Verification items for the finished model (mm, model axes). A direction names the side the tool comes from. Round coordinates to 2 decimals unless told otherwise and drop trailing zeros. Write each loop counter-clockwise with the first axis right and the second up, starting at its lowest first coordinate (ties: lowest second). Pieces come first, ordered by that corner, then holes. Notation, with made-up numbers: M -35.5,58 L -6.5,58 A25 ccw -6.5,94 Z; hole C 34,-19.75 d2. An arc over 180 degrees is marked long. One line per question, with ' | ' between items.
Autodesk Inventor part; units mm, degrees
ref_plane "YZ Plane" through (0, 0, 0) normal (1, 0, 0) x (0, 1, 0)
ref_plane "XZ Plane" through (0, 0, 0) normal (0, 1, 0) x (-1, 0, 0)
ref_plane "XY Plane" through (0, 0, 0) normal (0, 0, 1) x (1, 0, 0)
sketch "Esboço1" plane through (0, 0, 0) normal (0, 0, 1) x (1, 0, 0)
  line L0 (17.7277, 1.9549) -> (-24.2723, 1.9549)
  line L1 (-24.2723, 1.9549) -> (-24.2723, 7.9549)
  line L2 (17.7277, 7.9549) -> (17.7277, 1.9549)
  line L3 (6.7277, 39.4549) -> (6.7277, 7.9549)
  line L4 (-13.2723, 7.9549) -> (-13.2723, 39.4549)
  arc A0 (-4.2723, 30.871) -> (-2.2723, 30.871) centre (-3.2723, 24.9549) ccw
  line L5 (-24.2723, 7.9549) -> (-13.2723, 7.9549)
  line L6 (6.7277, 7.9549) -> (17.7277, 7.9549)
  line L7 (-2.2723, 39.4549) -> (-2.2723, 30.871)
  line L8 (-4.2723, 30.871) -> (-4.2723, 39.4549)
  line L9 (-13.2723, 39.4549) -> (-4.2723, 39.4549)
  line L10 (-2.2723, 39.4549) -> (6.7277, 39.4549)
  dimension "largura" = 42
  dimension "largura_topo" = 20
  dimension "altura_base" = 6
  dimension "diametro" = 12
  dimension "altura_furo" = 23
  dimension "d6" = 11
  dimension "d7" = 10
  dimension "d8" = 6
  dimension "d10" = 9
  dimension "d11" = 9
  dimension "altura" = 37.5
  dimension "d33" = 37.5
extrude "Extrusão1" add sketch "Esboço1" along normal blind 16
sketch "Esboço2" plane through (6.7277, 7.9549, 0) normal (1, 0, 0) x (0, 0, -1)
  line L0 (0, 22.9161) -> (-16, 22.9161)
  line L1 (-8, 22.9161) -> (-8, 31.5) construction
  circle A0 centre (-8, 27.208) radius 1.1711 construction
  line L2 (0, 31.5) -> (-16, 31.5)
  point P0 (0, -7.9549)
hole "Furo1" at (6.7277, 35.163, 8) direction (-1, 0, 0) diameter 3.242 end through all counterbore diameter 6 counterbore depth 4
sketch "Esboço3" plane through (-24.2723, 1.9549, 0) normal (0, -1, 0) x (1, 0, 0)
  line L0 (5, 8) -> (37, 8) construction
  circle A0 centre (5, 8) radius 1 construction
  circle A1 centre (37, 8) radius 1 construction
  line L1 (42, 0) -> (0, 0) construction
  line L2 (21, 0) -> (21, 16) construction
  line L3 (0, 16) -> (42, 16) construction
  point P0 (21, 8)
  dimension "distancia_parafusos" = 32
  dimension "d22" = 2
  dimension "d23" = 2
hole "Furo2" at (-19.2723, 1.9549, 8) at (12.7277, 1.9549, 8) direction (0, 1, 0) diameter 5.5 end through all
fillet "Arredondamento1" radius 1 4 edges at (6.7277, 39.4549, 8) (-13.2723, 39.4549, 8) (-24.2723, 7.9549, 8) (17.7277, 7.9549, 8)
equation "\"d6\" = -0.5 * largura_topo + 0.5 * largura"
equation "\"d7\" = 0.5 * largura_topo"
equation "\"d8\" = altura_base"
equation "\"d11\" = d10"
equation "\"d33\" = altura"
properties part number "Sk12"
1. Section check C-C, the plane z = 4.5. Record the cut outline in (x, y).
Results:
outline: M -24.27,1.95 L 17.73,1.95 L 17.73,6.95 A1 ccw 16.73,7.95 L 6.73,7.95 L 6.73,38.45 A1 ccw 5.73,39.45 L -2.27,39.45 L -2.27,30.87 A6 cw long -4.27,30.87 L -4.27,39.45 L -12.27,39.45 A1 ccw -13.27,38.45 L -13.27,7.95 L -23.27,7.95 A1 ccw -24.27,6.95 Z
2. Tool access check on faces 1 (the face through (-2.272, 35, 6)), 2 (the face through (6.728, 23, 8)), 3 (the face through (4.7, 34.26, 5.14)). Record the directions out of +Z, -Z, +X, -X, +Y, -Y that give a thin tool (end or side, any length) a straight path to the whole face; none if there is none.
Results:
face 1: +Z, -Z, +Y | face 2: +Z, -Z, +X, +Y | face 3: +X
3. Go/stop test with flat-tipped pins: P1, Ø6, axis at y = 10, z = 6, coming from the -X side; P2, Ø3, axis at y = 33.5, z = 6.5, coming from the +X side; P3, Ø5.5, axis at y = 35.163, z = 8, coming from the +X side; P4, Ø4.5, axis at y = 36, z = 4, coming from the -X side. Record where each tip stops, or that it passes through.
Results:
P1: stops at x = -24.27 | P2: stops at x = 6.73 | P3: stops at x = 2.73 | P4: stops at x = -13.27
4. Section check B-B, the plane y = 21.5. Record the cut outline in (x, z).
Results:
outline: M -13.27,0 L -8.18,0 L -8.18,16 L -13.27,16 Z; M 1.63,0 L 6.73,0 L 6.73,16 L 1.63,16 Z
5. Section check D-D, the plane x = 11. Record the cut outline in (y, z).
Results:
outline: M 1.95,0 L 7.95,0 L 7.95,5.86 L 1.95,5.86 Z; M 1.95,10.14 L 7.95,10.14 L 7.95,16 L 1.95,16 Z
6. Thickness scan on line 1 (X direction, y = 6.25, z = 8); line 2 (X direction, y = 31, z = 7); line 3 (X direction, y = 32.5, z = 7.75). Record the ranges inside material, lowest first.
Results:
line 1: x = -24.27 to -22.02, -16.52 to 9.98, 15.48 to 17.73 | line 2: x = -13.27 to -4.27, -2.27 to 6.73 | line 3: x = -13.27 to -4.27, -2.27 to 2.73
7. Mould release check, pull along X, two halves, no side actions. Record for faces 4 (the face through (-23.97, 7.67, 8.11)), 5 (the face through (-4, 17, 16)), 6 (the face through (-3.02, 18.96, 7.89)), 7 (the face through (-22, 5, 8.36)): pulls with the +X half, pulls with the -X half, needs draft (parallel to the pull), parting line crosses it, or undercut.
Results:
face 4: pulls with the -X half | face 5: needs draft | face 6: undercut | face 7: undercut
8. Section check A-A, the plane x = 0.5. Record the cut outline in (y, z).
Results:
outline: M 1.95,0 L 20.29,0 L 20.29,16 L 1.95,16 Z; M 29.62,0 L 39.45,0 L 39.45,16 L 29.62,16 Z; hole C 35.16,8 d3.24
